```python
from build123d import *

# Parameters (mm, degrees)
F0_W     = 300
F0_H     = 170
F1_DEPTH = 5


with BuildPart() as f1:
    # F0 (on Top) → F1 (new body)
    with BuildSketch(Plane.XY):
        Polygon((600, 0), (0, 0), (0, -100), (150, -100), (150, -200), (0, -200), (0, -400), (150, -400), (450, -400), (600, -400), (600, -200), (450, -200), (450, -100), (600, -100), align=None)
        with Locations((300, -485)):
            Rectangle(F0_W, F0_H)
    extrude(amount=F1_DEPTH)


solid = f1.part
```
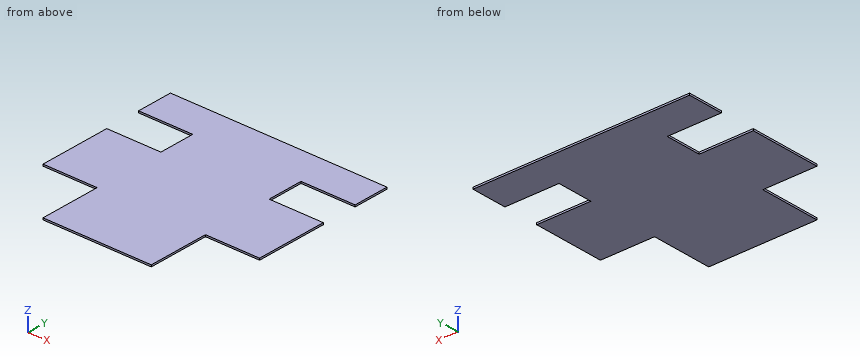
Check sheet for the modelled part. Datum: model origin and axes. Units: mm. Coordinates: 2 decimals unless noted, no trailing zeros. Loops run counter-clockwise (first coordinate to the right, second up) from the corner with the lowest first, then second, coordinate; pieces in that order, holes last.
1) Gauge pin test, flat ends, axial feed: pin 1 (2.5 mm diameter, centred on y = -501.5, z = 3.5, fed in from -X); pin 2 (1.5 mm diameter, centred on x = 99, z = 3.5, fed in from -Y); pin 3 (6 mm diameter, centred on x = 278, y = -76.5, fed in from -Z). Record the tip position at first contact, or that the pin passes through.
2) Sectioned sample at A-A (x = 115.5). Record the boundary of the cut face in (y, z), and give its area (3 significant figures).
3) Sectioned sample at B-B (z = 2.5). Record the boundary of the cut face in (x, y), and give its area (3 significant figures).
4) Sectioned sample at C-C (y = -115). Record the boundary of the cut face in (x, z), and give its area (3 significant figures).
5) Material ranges on probe 1 along Y at (x, z) = (562.5, 3.05); probe 2 along X at (y, z) = (-483.5, 3.75), recorded low to high.
Check sheet entries:
1. pin 1: stops at x = 150
1. pin 2: stops at y = -400
1. pin 3: stops at z = 0
2. outline: (-400, 0) - (-200, 0) - (-200, 5) - (-400, 5) - close; (-100, 0) - (0, 0) - (0, 5) - (-100, 5) - close
2. area: 1,500 mm2
3. outline: (0, -400) - (150, -400) - (150, -570) - (450, -570) - (450, -400) - (600, -400) - (600, -200) - (450, -200) - (450, -100) - (600, -100) - (600, 0) - (0, 0) - (0, -100) - (150, -100) - (150, -200) - (0, -200) - close
3. area: 261,000 mm2
4. outline: (150, 0) - (450, 0) - (450, 5) - (150, 5) - close
4. area: 1,500 mm2
5. probe 1: y = -400 to -200, -100 to 0
5. probe 2: x = 150 to 450
